```python
from build123d import *

# Parameters (mm, degrees)
BOSS_EXTRUDE1_DEPTH     = 6.75
SKETCH2_R               = 0.5
CUT_EXTRUDE1_DEPTH      = 3.5
CUT_EXTRUDE1_DEPTH_BACK = 3


with BuildPart() as part:
    # Sketch1 → Boss-Extrude1 (new body)
    with BuildSketch(Plane.XY):
        Polygon((37.296734757, 0.25), (47.546734757, 0.25), (59.223236254, -2.25), (110.463879182, -2.25), (122.14020427, 0.25), (126.893469513, 0.25), (126.893469513, 2.25), (122.178494939, 2.25), (110.502169851, -0.25), (59.684942458, -0.25), (48.00844096, 2.25), (37.085028553, 2.25), (25.408527056, -0.25), (-25.408700338, -0.25), (-37.085025426, 2.25), (-42.05, 2.25), (-42.05, 0.25), (-37.296734757, 0.25), (-25.620409669, -2.25), (25.620233259, -2.25), align=None)
    extrude(amount=BOSS_EXTRUDE1_DEPTH)

    # Sketch2 → Cut-Extrude1 (cut, two sides)
    with BuildSketch(Plane(origin=(0, -0.25, 0), x_dir=(1, 0, 0), z_dir=(0, 1, 0))) as cut_extrude1_sk:
        with Locations((45.113142199, -3.760486085)):
            Circle(SKETCH2_R)
        with Locations((65.993568392, -2.514696302)):
            Circle(SKETCH2_R)
        with Locations((103.888971043, -2.514696302)):
            Circle(SKETCH2_R)
        with Locations((124.713142199, -3.760486085)):
            Circle(SKETCH2_R)
        with Locations((39.863142199, -3.760486085)):
            Circle(SKETCH2_R)
        with Locations((-39.736857801, -3.760486085)):
            Circle(SKETCH2_R)
        with Locations((19.038971043, -2.514696302)):
            Circle(SKETCH2_R)
        with Locations((-18.856431608, -2.514696302)):
            Circle(SKETCH2_R)
    extrude(amount=CUT_EXTRUDE1_DEPTH, mode=Mode.SUBTRACT)
    extrude(cut_extrude1_sk.sketch, amount=-CUT_EXTRUDE1_DEPTH_BACK, mode=Mode.SUBTRACT)


solid = part.part
```
The listing builds one solid part. Answer for the finished solid, in the listing's coordinates (mm). A direction names the side the tool comes from. Give positions to 0.01 mm unless a question says otherwise; leave off trailing zeros. Write each loop counter-clockwise with the first axis right and the second up, starting at its lowest first coordinate (ties: lowest second). Pieces come first, ordered by that corner, then holes. Notation, with made-up numbers: (45.5, 5.5) -> (62.5, 5.5) arc R28 cw to (62.5, 24.5) -> close; hole circle Ø10 at (-39.5, -28.75). An arc over 180 degrees is marked (long way). Write item = value, one per line. Start each with the question number.
1) Straight lines are drawn through the part: line 1 along Y through (x, z) = (110, 1.25); line 2 along Y through (x, z) = (44, 2.5). For each, find the intervals that lie inside material, in ascending order.
2) Which of the six approach directions +Z, -Z, +X, -X, +Y, -Y give full straight-line access (tool end or side, diameter ignored) to faces 5 (the face through (116.422, 1.017, 3.328)), 6 (the face through (124, 0.25, 3)), 7 (the face through (42, 0.25, 3))?
3) The part is cut by section A-A, the plane y = 1.05. Determine the outline of the cut face in (x, z).
4) The part is cut by section C-C, the plane x = -0.5. Determine the outline of the cut face in (y, z), and give its area (3 significant figures).
5) The part is cut by section B-B, the plane z = 5.5. Determine the outline of the cut face in (x, y), and give its area (3 significant figures).
6) The part is cut by section D-D, the plane x = -30.5. Determine the outline of the cut face in (y, z).
7) Determine the mould class of faces 1 (the face through (116.22, -1.017, 3.328)), 2 (the face through (-39, 0.25, 3)), 3 (the face through (-31.54, -0.983, 3.328)), 4 (the face through (-31.165, 0.983, 3.328)) for opening direction X: +X half, -X half, draft (parallel to the pull), parting line (faces both ways), or undercut.
8) Each of these flat-tipped pins is pushed along its axis until it touches: pin 1 (1.4 mm diameter, centred on x = 124.5, z = 2.5, fed in from -Y); pin 2 (2 mm diameter, centred on x = 79.5, y = -1, fed in from -Z); pin 3 (2 mm diameter, centred on x = 77.5, z = 4.5, fed in from +Y). Where does it stop, or does it pass through?
Solutions:
q1.line_1 = -2.25 to -0.25
q1.line_2 = 0.25 to 2.25
q2.face_5 = +Z, -Z, +Y
q2.face_6 = +Z, -Z, +X, -Y
q2.face_7 = +Z, -Z, -Y
q3.outline = (-42.05, 0) -> (-31.48, 0) -> (-31.48, 6.75) -> (-42.05, 6.75) -> close; (31.48, 0) -> (53.61, 0) -> (53.61, 6.75) -> (31.48, 6.75) -> close; (116.57, 0) -> (126.89, 0) -> (126.89, 6.75) -> (116.57, 6.75) -> close; hole circle Ø1 at (-39.74, 3.76); hole circle Ø1 at (39.86, 3.76); hole circle Ø1 at (45.11, 3.76); hole circle Ø1 at (124.71, 3.76)
q4.outline = (-2.25, 0) -> (-0.25, 0) -> (-0.25, 6.75) -> (-2.25, 6.75) -> close
q4.area = 13.5 mm²
q5.outline = (-42.05, 0.25) -> (-37.3, 0.25) -> (-25.62, -2.25) -> (25.62, -2.25) -> (37.3, 0.25) -> (47.55, 0.25) -> (59.22, -2.25) -> (110.46, -2.25) -> (122.14, 0.25) -> (126.89, 0.25) -> (126.89, 2.25) -> (122.18, 2.25) -> (110.5, -0.25) -> (59.68, -0.25) -> (48.01, 2.25) -> (37.09, 2.25) -> (25.41, -0.25) -> (-25.41, -0.25) -> (-37.09, 2.25) -> (-42.05, 2.25) -> close
q5.area = 340 mm²
q6.outline = (-1.21, 0) -> (0.84, 0) -> (0.84, 6.75) -> (-1.21, 6.75) -> close
q7.face_1 = +X half
q7.face_2 = draft
q7.face_3 = -X half
q7.face_4 = undercut
q8.pin_1 = 0.25
q8.pin_2 = 0
q8.pin_3 = -0.25
